```python
from build123d import *

# Parameters (mm, degrees)
BOSS_EXTRUDE1_DEPTH = 3
BOSS_EXTRUDE1_TAPER = 10
BOSS_EXTRUDE2_DEPTH = 2
BOSS_EXTRUDE2_TAPER = 10


with BuildPart() as part:
    # Sketch2 → Boss-Extrude1 (new body)
    with BuildSketch(Plane(origin=(0, 0, 0), x_dir=(1, 0, 0), z_dir=(0, 1, 0))):
        Polygon((-1.528324253, 5.492415284), (-3.355149336, 3.355149336), (-6.507318108, 3.761110466), (-3.964091031, 0), (-3.964091031, -3.748296105), (-1.528324253, -3.748296105), (-1.002962791, -6.352097676), (1.719364784, -6.352097676), (3.916975027, -8.077462319), (6.642811529, -6.642811529), (7.116259803, -4.393932227), (3.534249835, -4.393932227), (2.579047177, -2.579047177), (3.534249835, -0.955202658), (-1.002962791, 0), align=None)
    extrude(amount=BOSS_EXTRUDE1_DEPTH, taper=BOSS_EXTRUDE1_TAPER)

    # Sketch3 → Boss-Extrude2 (add)
    with BuildSketch(Plane(origin=(0, 0, 0), x_dir=(1, 0, 0), z_dir=(0, 1, 0))):
        Polygon((10.386967226, -14.630930723), (9.354403277, -7.948617551), (7.630259288, -9.221195787), (7.015272692, -5.241265011), (4.708870367, -5.597654757), (5.613726928, -12.562233064), (8.245836253, -11.251331436), align=None)
        Polygon((3.707378368, -5.391000258), (1.988983683, -4.390600081), (-2.180835877, -10.285076618), (-0.270036733, -10.483558335), (-2.891449297, -14.630930723), (3.003431491, -9.596279278), (1.427179104, -9.307715176), align=None)
        Polygon((-11.789266005, -15.483155877), (-5.37466541, -12.099434913), (-7.404660906, -10.285076618), (-3.889999551, -8.299445569), (-3.889999551, -5.68241554), (1.090991617, -4.01155513), (-0.815187592, -0.637527311), (-6.297024016, -3.52921239), (-10.680628975, -1.975898906), (-10.680628975, -4.390600081), (-15.742910277, -2.79186121), (-9.511821995, -6.730319487), (-8.455251073, -4.981182544), (-6.701594742, -7.03447166), (-11.179985311, -11.251331436), (-8.967737144, -11.949990188), align=None)
        Polygon((-15.639992384, 10.338429497), (-13.782364953, 3.575498575), (-10.680628975, 4.134580902), (-8.967737144, 0.485871688), (-1.660461726, 0), (-3.965321164, 2.653546974), (-6.995301565, 3.038510834), (-10.680628975, 8.413901489), (-13.040069267, 6.586416727), align=None)
    extrude(amount=BOSS_EXTRUDE2_DEPTH, taper=BOSS_EXTRUDE2_TAPER)


solid = part.part
```
Part model, mm, in its own coordinate system. A direction names the side the tool comes from. Give positions to 0.01 mm unless a question says otherwise; leave off trailing zeros. Return JSON: item names as keys, results as strings.
1) 3-axis set-ups, long thin cutter, end or side, ignore diameter. For faces 1 (the face through (7, 2, 10)), 2 (the face through (-6, 2, 7)), 3 (the face through (0, 3, 2)): which of +Z, -Z, +X, -X, +Y, -Y reach the whole face in a straight line?
Calculated:
{"face 1": "+Z, +X, +Y", "face 2": "+Z, -X, +Y", "face 3": "+Z, -Z, +X, -X, +Y"}
2) Drill centre lines: line 1 (X direction, y = 0.2, z = 13.5); line 2 (Z direction, x = -6, y = 1.5); line 3 (Z direction, x = -13, y = 0.5). Where is each one in solid material? Low to high.
Calculated:
{"line 1": "x = -10.16 to -8.11, -2.13 to -1.62, 9.71 to 10.18", "line 2": "z = -2.65 to -0.55, 3.67 to 9.19, 11.9 to 12.13", "line 3": "z = -6.51 to -3.81, 3.75 to 4.42"}
3) Flat gauge pin, fed straight in: pin 1 Ø4.5 at (x, z) = (0.5, 10.5) entering from +Y. Where does the tip first touch, or does it go through?
Calculated:
{"pin 1": "stops at y = 2"}
